Model file for the job. Use its own axes, mm. A direction names the side the tool comes from. Round coordinates to 2 decimals unless told otherwise and drop trailing zeros. Loops run counter-clockwise (first coordinate to the right, second up) from the corner with the lowest first, then second, coordinate; pieces in that order, holes last. Notation, with made-up numbers: M 8,11 L 31,11 A5 cw 31,18 Z; hole C 61,49.5 d10. An arc over 180 degrees is marked long. Use a Markdown table: item, result. Add a question column.
Item 1: Two-plate mould, pull along Y, no slides. Class faces 6 (the flat face through (-23.2, -122.51, 28.64)), 7 (the flat face through (38, -9.482, 27)), 8 (the flat face through (96.053, -66, 46)): +Y half, -Y half, draft (parallel to the pull), parting line (faces both ways), or undercut.
Item 2: Pin check, flat tips, straight feed: P1, Ø12, axis at x = 0.5, z = 19.5, coming from the +Y side; P2, Ø1, axis at x = -18.5, y = -51.5, coming from the -Z side; P3, Ø0.9, axis at x = -98.5, z = 52, coming from the -Y side; P4, Ø3, axis at x = -14, y = -122, coming from the -Z side. Stop position of each tip, or through.
Item 3: Saw through at C-C on x = -44. Write the cut outline in (y, z).
Item 4: Tool access for faces 1 (the flat face through (46, -66, 3)), 2 (the flat face through (-18, -120.482, 26)), 3 (the flat face through (-23, -123, 49)), 4 (the flat face through (62, -12.482, 27)), 5 (the cylindrical face through (39.36, -41.82, 1.48)): list every direction of +Z, -Z, +X, -X, +Y, -Y with a clear straight run to the whole face (end or side of a thin tool).
Item 5: Wall check: L1, parallel to Z at x = 37, y = -39; L2, parallel to Y at x = 48, z = 31; L3, parallel to Y at x = -60.5, z = 43. Give the ranges that are in metal, low to high. Write a range as from..to.
Item 6: Saw through at B-B on z = 21. Write the cut outline in (x, y), then the cut area to 3 significant figures.
Item 7: Saw through at D-D on x = 71. Write the cut outline in (y, z), then the cut area to 3 significant figures.
Item 8: Saw through at A-A on y = -61. Write the cut outline in (x, z), then the cut area to 3 significant figures.
```python
from build123d import *

# Parameters (mm, degrees)
SKETCH_2_W          = 76
SKETCH_2_H          = 115
SKETCH_2_R          = 2.2
SKETCH_2_R_2        = 1.6
EXTRUDE_1_DEPTH     = 3
EXTRUDE_2_DEPTH     = 76
SKETCH_4_W          = 47
SKETCH_4_H          = 108.999999999
EXTRUDE_3_DEPTH     = 3
SKETCH_5_W          = 12
SKETCH_5_H          = 115
SKETCH_5_R          = 1.6
EXTRUDE_4_DEPTH     = 3
FILLET_1_R          = 2
SKETCH_6_W          = 3
SKETCH_6_H          = 115
EXTRUDE_5_DEPTH     = 110
SKETCH_7_R          = 1.6
CUT_EXTRUDE_1_DEPTH = 110
SKETCH_8_W          = 31
SKETCH_8_H          = 65
CUT_EXTRUDE_2_DEPTH = 3
EXTRUDE_6_DEPTH     = 4
EXTRUDE_7_DEPTH     = 4
CUT_EXTRUDE_3_DEPTH = 124
SKETCH_16_W         = 3
SKETCH_16_H         = 40
EXTRUDE_10_DEPTH    = 40
SKETCH_17_R         = 1.05
CUT_EXTRUDE_5_DEPTH = 40
FILLET_5_R          = 2
SKETCH_18_W         = 22
SKETCH_18_H         = 87
CUT_EXTRUDE_6_DEPTH = 4


with BuildPart() as part:
    # 草图2 → 凸台-拉伸1 (new body)
    with BuildSketch(Plane.XY):
        with Locations((61.052848474, -66.98174403)):
            Rectangle(SKETCH_2_W, SKETCH_2_H)
        with Locations((86.052848474, -91.272111932)):
            Circle(SKETCH_2_R, mode=Mode.SUBTRACT)
        with Locations((86.052848474, -42.48174403)):
            Circle(SKETCH_2_R, mode=Mode.SUBTRACT)
        with Locations((37.262480572, -42.48174403)):
            Circle(SKETCH_2_R, mode=Mode.SUBTRACT)
        with Locations((37.262480572, -91.272111932)):
            Circle(SKETCH_2_R, mode=Mode.SUBTRACT)
        with Locations((89.052848474, -16.98174403)):
            Circle(SKETCH_2_R_2, mode=Mode.SUBTRACT)
        with Locations((79.052848474, -16.98174403)):
            Circle(SKETCH_2_R_2, mode=Mode.SUBTRACT)
        with Locations((41.052848474, -16.98174403)):
            Circle(SKETCH_2_R_2, mode=Mode.SUBTRACT)
        with Locations((51.052848474, -16.98174403)):
            Circle(SKETCH_2_R_2, mode=Mode.SUBTRACT)
        with Locations((41.052848474, -116.98174403)):
            Circle(SKETCH_2_R_2, mode=Mode.SUBTRACT)
        with Locations((51.052848474, -116.98174403)):
            Circle(SKETCH_2_R_2, mode=Mode.SUBTRACT)
        with Locations((79.052848474, -116.98174403)):
            Circle(SKETCH_2_R_2, mode=Mode.SUBTRACT)
        with Locations((89.052848474, -116.98174403)):
            Circle(SKETCH_2_R_2, mode=Mode.SUBTRACT)
    extrude(amount=EXTRUDE_1_DEPTH)

    # 草图3 → 凸台-拉伸2 (add)
    with BuildSketch(Plane.ZY.offset(-23.052848474)):
        Polygon((0, -9.48174403), (53, -9.48174403), (53, -124.48174403), (0, -124.48174403), (0, -121.48174403), (50, -121.48174403), (50, -12.481744031), (0, -12.481744031), align=None)
    extrude(amount=-EXTRUDE_2_DEPTH)

    # 草图4 → 凸台-拉伸3 (add)
    with BuildSketch(Plane.ZY.offset(-23.052848474)):
        with Locations((26.5, -66.98174403)):
            Rectangle(SKETCH_4_W, SKETCH_4_H)
    extrude(amount=-EXTRUDE_3_DEPTH)

    # 草图5 → 凸台-拉伸4 (add)
    with BuildSketch(Plane(origin=(99.052848474, 0, 0), x_dir=(0, 0, -1), z_dir=(1, 0, 0))):
        with Locations((-47, -66.98174403)):
            Rectangle(SKETCH_5_W, SKETCH_5_H)
        with Locations(Location((-46, -117.48174403, 0), (0, 0, 90))):
            Circle(SKETCH_5_R, mode=Mode.SUBTRACT)
        with Locations(Location((-46, -16.48174403, 0), (0, 0, 90))):
            Circle(SKETCH_5_R, mode=Mode.SUBTRACT)
    extrude(amount=-EXTRUDE_4_DEPTH)

    # 圆角1
    fillet_1_edges = [part.edges().sort_by_distance(p)[0] for p in [
        (62.552848474, -12.481744031, 3),
        (61.052848474, -12.481744031, 50),
        (61.052848474, -121.48174403, 50),
        (97.552848474, -121.48174403, 41),
        (97.552848474, -12.481744031, 41),
        (61.052848474, -9.48174403, 0),
        (61.052848474, -124.48174403, 0),
        (62.552848474, -121.48174403, 3),
    ]]
    fillet(fillet_1_edges, radius=FILLET_1_R)

    # 草图6 → 凸台-拉伸5 (add)
    with BuildSketch(Plane.ZY.offset(-23.052848474)):
        with Locations((51.5, -66.98174403)):
            Rectangle(SKETCH_6_W, SKETCH_6_H)
    extrude(amount=EXTRUDE_5_DEPTH)

    # 草图7 → 切除-拉伸1 (cut)
    with BuildSketch(Plane(origin=(0, 0, 50), x_dir=(-1, 0, 0), z_dir=(0, 0, -1))):
        with Locations(Location((81.947151526, -21.98174403, 0), (0, 0, 90))):
            Circle(SKETCH_7_R)
        with Locations(Location((81.947151526, -111.98174403, 0), (0, 0, 90))):
            Circle(SKETCH_7_R)
        with Locations(Location((-8.052848474, -21.98174403, 0), (0, 0, 90))):
            Circle(SKETCH_7_R)
        with Locations(Location((-8.052848474, -111.98174403, 0), (0, 0, 90))):
            Circle(SKETCH_7_R)
    extrude(amount=-CUT_EXTRUDE_1_DEPTH, mode=Mode.SUBTRACT)

    # 草图8 → 切除-拉伸2 (cut)
    with BuildSketch(Plane(origin=(0, 0, 0), x_dir=(-1, 0, 0), z_dir=(0, 0, -1))):
        with Locations((-63.552848474, -66.98174403)):
            Rectangle(SKETCH_8_W, SKETCH_8_H)
    extrude(amount=-CUT_EXTRUDE_2_DEPTH, mode=Mode.SUBTRACT)

    # 草图9 → 凸台-拉伸6 (add)
    with BuildSketch(Plane(origin=(0, -124.48174403, 0), x_dir=(-1, 0, 0), z_dir=(0, -1, 0))):
        Polygon((-23.052848474, -2), (81.947151526, -50), (-23.052848474, -50), align=None)
    extrude(amount=-EXTRUDE_6_DEPTH)

    # 草图10 → 凸台-拉伸7 (add)
    with BuildSketch(Plane(origin=(0, -9.48174403, 0), x_dir=(1, 0, 0), z_dir=(0, 1, 0))):
        Polygon((23.052848474, -2), (-81.947151526, -50), (23.052848474, -50), align=None)
    extrude(amount=-EXTRUDE_7_DEPTH)

    # 草图11 → 切除-拉伸3 (cut)
    with BuildSketch(Plane(origin=(0, -124.48174403, 0), x_dir=(-1, 0, 0), z_dir=(0, -1, 0))):
        with BuildLine():
            Line((58.548005297, -49), (-14.052848474, -49))
            ThreePointArc((-14.052848474, -49), (-17.58838238, -47.535533906), (-19.052848474, -44))
            Line((-19.052848474, -44), (-19.052848474, -17.109646517))
            ThreePointArc((-19.052848474, -17.109646517), (-16.755255364, -12.902866632), (-11.974049673, -12.562274139))
            Line((-11.974049673, -12.562274139), (59.379524817, -45.181051049))
            ThreePointArc((59.379524817, -45.181051049), (60.502218425, -47.425500939), (58.548005297, -49))
        make_face()
    extrude(amount=-CUT_EXTRUDE_3_DEPTH, mode=Mode.SUBTRACT)

    # 草图16 → 凸台-拉伸10 (add)
    with BuildSketch(Plane.ZY.offset(86.947151526)):
        with Locations((51.5, -29.48174403)):
            Rectangle(SKETCH_16_W, SKETCH_16_H)
    extrude(amount=EXTRUDE_10_DEPTH)

    # 草图17 → 切除-拉伸5 (cut)
    with BuildSketch(Plane(origin=(0, 0, 50), x_dir=(-1, 0, 0), z_dir=(0, 0, -1))):
        with Locations(Location((121.947151526, -44.48174403, 0), (0, 0, 90))):
            Circle(SKETCH_17_R)
        with Locations(Location((121.947151526, -19.88174403, 0), (0, 0, 90))):
            Circle(SKETCH_17_R)
        with Locations(Location((97.347151526, -19.88174403, 0), (0, 0, 90))):
            Circle(SKETCH_17_R)
        with Locations(Location((97.347151526, -44.48174403, 0), (0, 0, 90))):
            Circle(SKETCH_17_R)
    extrude(amount=-CUT_EXTRUDE_5_DEPTH, mode=Mode.SUBTRACT)

    # 圆角5
    fillet_5_edges = [part.edges().sort_by_distance(p)[0] for p in [
        (-86.947151526, -124.48174403, 51.5),
        (-86.947151526, -49.48174403, 51.5),
        (-126.947151526, -49.48174403, 51.5),
        (-126.947151526, -9.48174403, 51.5),
    ]]
    fillet(fillet_5_edges, radius=FILLET_5_R)

    # 草图18 → 切除-拉伸6 (cut)
    with BuildSketch(Plane.ZY.offset(-23.052848474)):
        with Locations((19, -66.98174403)):
            Rectangle(SKETCH_18_W, SKETCH_18_H)
    extrude(amount=-CUT_EXTRUDE_6_DEPTH, mode=Mode.SUBTRACT)


solid = part.part
```
Entries:
| question | item | result |
|---|---|---|
| 1 | face 6 | draft |
| 1 | face 7 | +Y half |
| 1 | face 8 | undercut |
| 2 | P1 | y = -9.48 |
| 2 | P2 | z = 50 |
| 2 | P3 | y = -49.48 |
| 2 | P4 | z = 18.25 |
| 3 | outline | M -124.48,32.65 L -120.48,32.65 L -120.48,38.15 L -124.48,38.15 Z; M -124.48,49 L -120.48,49 L -120.48,50 L -13.48,50 L -13.48,49 L -9.48,49 L -9.48,53 L -124.48,53 Z; M -13.48,32.65 L -9.48,32.65 L -9.48,38.15 L -13.48,38.15 Z |
| 4 | face 1 | +X |
| 4 | face 2 | -Z, -X |
| 4 | face 3 | +Y, -Y |
| 4 | face 4 | none |
| 4 | face 5 | -Z |
| 5 | L1 | 0..3, 50..53 |
| 5 | L2 | -124.48..-121.48, -12.48..-9.48 |
| 5 | L3 | -124.48..-120.48, -13.48..-9.48 |
| 6 | outline | M -18.51,-124.48 L -6.48,-124.48 L -6.48,-120.48 L -18.51,-120.48 Z; M -18.51,-13.48 L -6.48,-13.48 L -6.48,-9.48 L -18.51,-9.48 Z; M 19.05,-124.48 L 99.05,-124.48 L 99.05,-121.48 L 26.05,-121.48 L 26.05,-110.48 L 23.05,-110.48 L 23.05,-120.48 L 19.05,-120.48 Z; M 19.05,-13.48 L 23.05,-13.48 L 23.05,-23.48 L 26.05,-23.48 L 26.05,-12.48 L 99.05,-12.48 L 99.05,-9.48 L 19.05,-9.48 Z |
| 6 | area | 650 mm2 |
| 7 | outline | M -124.48,2 A2 ccw -122.48,0 L -99.48,0 L -99.48,3 L -119.48,3 A2 cw -121.48,5 L -121.48,48 A2 cw -119.48,50 L -14.48,50 A2 cw -12.48,48 L -12.48,5 A2 cw -14.48,3 L -34.48,3 L -34.48,0 L -11.48,0 A2 ccw -9.48,2 L -9.48,53 L -124.48,53 Z |
| 7 | area | 779 mm2 |
| 8 | outline | M -86.95,50 L 23.05,50 L 23.05,30 L 26.05,30 L 26.05,50 L 96.05,50 L 96.05,41 L 99.05,41 L 99.05,53 L -86.95,53 Z; M 23.05,0 L 48.05,0 L 48.05,3 L 26.05,3 L 26.05,8 L 23.05,8 Z; M 79.05,0 L 99.05,0 L 99.05,3 L 79.05,3 Z |
| 8 | area | 795 mm2 |
